The figure shows three views and two pictorial views of one solid part (mm, origin at its lowest corner). Answer the questions. Coordinates: 2 decimals unless noted, no trailing zeros. Loops run counter-clockwise (first coordinate to the right, second up) from the corner with the lowest first, then second, coordinate; pieces in that order, holes last. Notation, with made-up numbers: M -29.75,-25 L 24.25,-25 A9 ccw 24.25,-12 Z; hole C 46.25,81.25 d6. An arc over 180 degrees is marked long. Write each question's results on one line, items separated by ' | '.
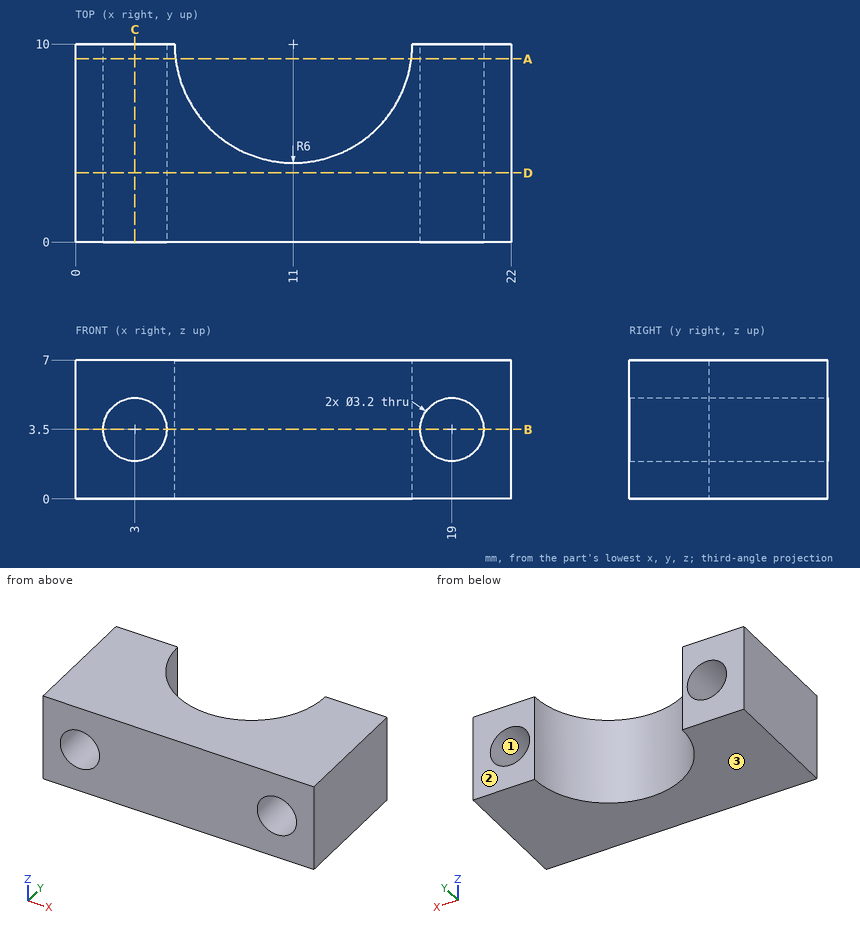
1) For a pull along Z with two mould halves and no side action, classify the marked faces 1, 2 and 3 as released by +Z, released by -Z, zero draft, split by the parting line, or undercut.
Check result:
face 1: undercut | face 2: zero draft | face 3: released by -Z
2) Find section C-C, the plane x = 3. Give the vertices of the cut face in (y, z), and give its area (3 significant figures).
Check result:
outline: M 0,0 L 10,0 L 10,1.9 L 0,1.9 Z; M 0,5.1 L 10,5.1 L 10,7 L 0,7 Z | area: 38.0 mm^2
3) Find section B-B, the plane z = 3.5. Give the vertices of the cut face in (x, y).
Check result:
outline: M 0,0 L 1.4,0 L 1.4,10 L 0,10 Z; M 4.6,0 L 17.4,0 L 17.4,10 L 17,10 A6 cw 5,10 L 4.6,10 Z; M 20.6,0 L 22,0 L 22,10 L 20.6,10 Z
4) Find section A-A, the plane y = 9.25. Give the vertices of the cut face in (x, z).
Check result:
outline: M 0,0 L 5.05,0 L 5.05,7 L 0,7 Z; M 16.95,0 L 22,0 L 22,7 L 16.95,7 Z; hole C 3,3.5 d3.2; hole C 19,3.5 d3.2
5) Find section D-D, the plane y = 3.5. Give the vertices of the cut face in (x, z), and give its area (3 significant figures).
Check result:
outline: M 0,0 L 22,0 L 22,7 L 0,7 Z; hole C 3,3.5 d3.2; hole C 19,3.5 d3.2 | area: 138 mm^2
6) Straight lines are drawn through the part: probe 1 along X at (y, z) = (3.25, 3.5); probe 2 along Z at (x, y) = (19, 6.5); probe 3 along X at (y, z) = (7.25, 2.75). For each, find the intervals that lie inside material, in ascending order. Write a range as [from, to].
Check result:
probe 1: [0, 1.4], [4.6, 17.4], [20.6, 22] | probe 2: [0, 1.9], [5.1, 7] | probe 3: [0, 1.59], [4.41, 5.67], [16.33, 17.59], [20.41, 22]
7) Given pin 1 Ø3 at (x, z) = (13.5, 6) entering from +Y, flat-ended and moving along its own axis, determine where the tip first touches the part or whether it passes through.
Check result:
pin 1: y = 5.53
